Check sheet for the modelled part. Datum: model origin and axes. Units: mm. Face numbers are marked on the shaded views. A direction names the side the tool comes from. Coordinates: 2 decimals unless noted, no trailing zeros. Loops run counter-clockwise (first coordinate to the right, second up) from the corner with the lowest first, then second, coordinate; pieces in that order, holes last.
```python
from build123d import *

# Parameters (mm, degrees)
SKETCH1_W          = 12
SKETCH1_H          = 3
SKETCH4_W          = 11
SKETCH4_H          = 11
CUT_EXTRUDE1_DEPTH = 2.4


with BuildPart() as part:
    # Sketch1 → Revolve1 (revolve)
    with BuildSketch(Plane(origin=(0, 0, 0), x_dir=(0, 0, -1), z_dir=(1, 0, 0)), mode=Mode.PRIVATE) as revolve1_sk:
        with Locations((0, 1.5)):
            Rectangle(SKETCH1_W, SKETCH1_H)
    revolve(revolve1_sk.sketch.rotate(Axis((0, 0, -6), (0, 0, 1)), 270), axis=Axis((0, 0, -6), (0, 0, 1)))

    # Sketch2 → Revolve2 (revolve)
    with BuildSketch(Plane.XY, mode=Mode.PRIVATE) as revolve2_sk:
        Polygon((-10, 0), (-10, 1.1935), (-9.6935, 1.5), (-2.8065, 1.5), (-2.5, 1.1935), (-2.5, 0), align=None)
    revolve(revolve2_sk.sketch.rotate(Axis((-2.5, 0, 0), (-1, 0, 0)), 270), axis=Axis((-2.5, 0, 0), (-1, 0, 0)))

    # Sketch3 → Revolve3 (revolve)
    with BuildSketch(Plane.XY, mode=Mode.PRIVATE) as revolve3_sk:
        Polygon((-9.9, 2.75), (-9.9, 1.5), (-7.5, 1.5), (-7.5, 2.75), (-7.654842576, 3.175426481), (-9.745157424, 3.175426481), align=None)
    revolve(revolve3_sk.sketch.rotate(Axis((42.5, 0, 0), (-1, 0, 0)), 270), axis=Axis((42.5, 0, 0), (-1, 0, 0)))

    # Sketch4 → Cut-Extrude1 (cut)
    with BuildSketch(Plane(origin=(-7.5, 0, 0), x_dir=(0, 0, -1), z_dir=(1, 0, 0))):
        Rectangle(SKETCH4_W, SKETCH4_H)
        Polygon((-2.75, -1.58771324), (0, -3.175426481), (2.75, -1.58771324), (2.75, 1.58771324), (0, 3.175426481), (-2.75, 1.58771324), align=None, mode=Mode.SUBTRACT)
    extrude(amount=-CUT_EXTRUDE1_DEPTH, mode=Mode.SUBTRACT)


solid = part.part
```
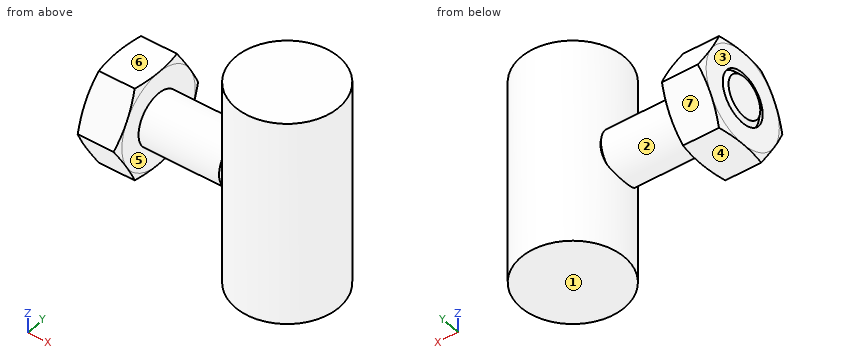
1) Mould release check, pull along X, two halves, no side actions. Record for the marked faces 1, 2 and 3: +X half, -X half, draft (parallel to the pull), parting line (faces both ways), or undercut.
Answer sheet:
face 1: draft
face 2: undercut
face 3: -X half
2) Scan lines: line 1 (X direction, y = -2.5, z = 0); line 2 (X direction, y = -0.75, z = -2.25); line 3 (Y direction, x = -1.5, z = -2.5). Record each from-to range of solid material in increasing order.
Answer sheet:
line 1: x = -9.9 to -7.5, -1.66 to 1.66
line 2: x = -9.9 to -7.5, -2.9 to 2.9
line 3: y = -2.6 to 2.6
3) Section check C-C on x = -5. Enter the section's corners in (y, z), plus the area to 3 significant figures.
Answer sheet:
outline: circle Ø3 at (0, 0)
area: 7.07 mm2
4) Section check D-D on x = -1.5. Enter the section's corners in (y, z).
Answer sheet:
outline: (-2.6, -6) - (2.6, -6) - (2.6, 6) - (-2.6, 6) - close
5) Depth check by flat-ended pin: pin 1 (2 mm diameter, centred on x = -3, y = 1, fed in from +Z); pin 2 (2.5 mm diameter, centred on x = -8.5, y = -0.5, fed in from +Z); pin 3 (1.2 mm diameter, centred on x = -9, y = 0, fed in from -Z); pin 4 (2 mm diameter, centred on x = -4.5, y = -0.5, fed in from -Z). Enter the tip coordinate at first touch or a pass-through.
Answer sheet:
pin 1: stops at z = 6
pin 2: stops at z = 2.75
pin 3: stops at z = -2.75
pin 4: stops at z = -1.5
6) Set-up check for the marked faces 4, 5, 6 and 7: record each of +Z, -Z, +X, -X, +Y, -Y from which the full face is reachable in a straight line by a thin tool's end or side.
Answer sheet:
face 4: -Z, -X, +Y, -Y
face 5: none
face 6: +Z, -X, +Y, -Y
face 7: -Z, -X, +Y
7) Section check A-A on x = 0. Enter the section's corners in (y, z).
Answer sheet:
outline: (-3, -6) - (3, -6) - (3, 6) - (-3, 6) - close
8) Section check B-B on z = 5.5. Enter the section's corners in (x, y).
Answer sheet:
outline: circle Ø6 at (0, 0)
